Verification items for the finished model (mm, model axes). A direction names the side the tool comes from. Coordinates: 2 decimals unless noted, no trailing zeros. Loops run counter-clockwise (first coordinate to the right, second up) from the corner with the lowest first, then second, coordinate; pieces in that order, holes last. Notation, with made-up numbers: M 79,88 L 131,88 A23 cw 131,102 Z; hole C 10,34 d8. An arc over 180 degrees is marked long. Write item = value, one per line. Start each with the question number.
Autodesk Inventor part; units mm, degrees
ref_plane "YZ Plane" through (0, 0, 0) normal (1, 0, 0) x (0, 1, 0)
ref_plane "XZ Plane" through (0, 0, 0) normal (0, 1, 0) x (-1, 0, 0)
ref_plane "XY Plane" through (0, 0, 0) normal (0, 0, 1) x (1, 0, 0)
sketch "Sketch1" plane through (0, 0, 0) normal (0, 1, 0) x (-1, 0, 0)
  circle A0 centre (0, 0) radius 26.67
  circle A1 centre (2.413, -14.8844) radius 0.6
  circle A2 centre (2.413, -14.8844) radius 4.0005
  circle A3 centre (14.8844, 2.413) radius 4.0005
  circle A4 centre (14.8844, 2.413) radius 0.6
  circle A5 centre (-2.413, 14.8844) radius 4.0005
  circle A6 centre (-2.413, 14.8844) radius 0.6
  circle A7 centre (-14.8844, -2.413) radius 4.0005
  circle A8 centre (-14.8844, -2.413) radius 0.6
  circle A9 centre (15.5194, -17.1704) radius 1.524
  circle A10 centre (17.1704, 15.5194) radius 1.524
  circle A11 centre (-15.5194, 17.1704) radius 1.524
  circle A12 centre (-17.1704, -15.5194) radius 1.524
  dimension "d0" = 53.34
  dimension "d7" = 360
  dimension "d14" = 360
extrude "Extrusion1" add sketch "Sketch1" against normal blind 10.0076 contours A0 | A2 | A3 | A5 | A7 | A8
hole "Hole1" at (-14.8844, 0, 2.413) direction (0, -1, 0) diameter 8 depth 7.493
hole "Hole2" at (-2.413, 0, -14.8844) at (2.413, 0, 14.8844) at (14.8844, 0, -2.413) direction (0, -1, 0) diameter 8 depth 7.493
hole "Hole3" at (14.8844, 0, -2.413) direction (0, -1, 0) diameter 1.2 end through all
thread "Thread1"
thread "Thread2"
thread "Thread3"
thread "Thread4"
thread "Thread5"
thread "Thread6"
thread "Thread7"
thread "Thread8"
Q1. Mould release check, pull along X, two halves, no side actions. Record for faces 3 (the face through (3.472, -4.934, 26.443)), 4 (the face through (0, -10.008, 0)), 5 (the face through (-2, -7.493, -14)): +X half, -X half, draft (parallel to the pull), parting line (faces both ways), or undercut.
Q2. Sectioned sample at D-D on z = 5.5. Record the cut outline in (x, y), plus the area to 3 significant figures.
Q3. Set-up check for faces 1 (the face through (-3, -9, -15)), 2 (the face through (2.24, -3.8, 10.89)): record each of +Z, -Z, +X, -X, +Y, -Y from which the full face is reachable in a straight line by a thin tool's end or side.
Q4. Scan lines: L1, parallel to X at y = -3, z = 15; L2, parallel to Z at x = 16.5, y = -5.5; L3, parallel to X at y = -3, z = 16. Record each from-to range of solid material in increasing order. Write a range as [from, to].
Q5. Sectioned sample at B-B on y = -5. Count the separate pieces of the cut face and the enclosed holes in it, plus the area to 3 significant figures.
Q6. Sectioned sample at A-A on z = 0. Record the cut outline in (x, y).
Q7. Gauge pin test, flat ends, axial feed: pin 1 (6.5 mm diameter, centred on x = -14.88, z = 2.41, fed in from +Y); pin 2 (2.5 mm diameter, centred on x = 15.52, z = 17.17, fed in from +Y); pin 3 (2 mm diameter, centred on y = -4, z = 1.5, fed in from -X); pin 4 (3 mm diameter, centred on x = -9.5, y = -6, fed in from +Z). Record the tip position at first contact, or that the pin passes through.
Q8. Sectioned sample at C-C on x = 0. Record the cut outline in (y, z), plus the area to 3 significant figures.
Solutions:
q1.face_3 = parting line
q1.face_4 = draft
q1.face_5 = undercut
q2.outline = M -26.1,-10.01 L 26.1,-10.01 L 26.1,0 L -12.34,0 L -12.34,-7.49 L -17.43,-7.49 L -17.43,0 L -26.1,0 Z
q2.area = 484 mm²
q3.face_1 = +Y, -Y
q3.face_2 = +Y
q4.L1 = [-22.05, -18.6], [-15.74, -1.59], [6.41, 22.05]
q4.L2 = [-20.95, -16.89], [-14.15, -6.07], [1.25, 16], [18.34, 20.95]
q4.L3 = [-21.34, -18.62], [-15.72, -1.43], [6.25, 14.54], [16.5, 21.34]
q5.separate_pieces = 1
q5.enclosed_holes = 8
q5.area = 2,000 mm²
q6.outline = M -26.67,-10.01 L 26.67,-10.01 L 26.67,0 L 18.07,0 L 18.07,-7.49 L 11.69,-7.49 L 11.69,0 L -11.69,0 L -11.69,-7.49 L -18.07,-7.49 L -18.07,0 L -26.67,0 Z
q7.pin_1 = -7.49
q7.pin_2 = through
q7.pin_3 = -26.67
q7.pin_4 = 25.44
q8.outline = M -10.01,-26.67 L 0,-26.67 L 0,-18.07 L -7.49,-18.07 L -7.49,-11.69 L 0,-11.69 L 0,11.69 L -7.49,11.69 L -7.49,18.07 L 0,18.07 L 0,26.67 L -10.01,26.67 Z
q8.area = 438 mm²
